Autodesk Inventor part; units mm, degrees
ref_plane "YZ Plane" through (0, 0, 0) normal (1, 0, 0) x (0, 1, 0)
ref_plane "XZ Plane" through (0, 0, 0) normal (0, 1, 0) x (-1, 0, 0)
ref_plane "XY Plane" through (0, 0, 0) normal (0, 0, 1) x (1, 0, 0)
sketch "Sketch1" plane through (0, 0, 0) normal (0, 1, 0) x (-1, 0, 0)
  line L0 (0, 0) -> (400, 0)
  line L1 (400, 0) -> (400, -100)
  line L2 (400, -100) -> (0, -100)
  line L3 (0, -100) -> (0, 0)
  line L4 (320, -103) -> (320, -100)
  line L5 (80, -103) -> (80, -100)
  line L6 (240, -100) -> (240, -103)
  line L7 (160, -103) -> (160, -100)
  line L8 (400, -25) -> (400, -50)
  line L9 (400, -50) -> (403, -50)
  line L10 (200, 0) -> (200, -100) construction
  line L11 (0, 0) -> (0, -100)
  line L12 (-3, -25) -> (0, -25)
  line L13 (0, -25) -> (0, -50)
  line L14 (0, -50) -> (-3, -50)
  line L15 (-3, -75) -> (0, -75)
  line L16 (320, -103) -> (240, -103)
  line L17 (160, -103) -> (80, -103)
  line L18 (0, -100) -> (-3, -100)
  line L19 (-3, -100) -> (-3, -75)
  line L20 (-3, -50) -> (-3, -25)
  line L21 (400, 0) -> (0, 0)
  line L22 (400, -100) -> (400, 0)
  line L23 (403, -75) -> (400, -75)
  line L24 (400, -50) -> (403, -50)
  line L25 (400, -25) -> (400, -50)
  line L26 (403, -25) -> (400, -25)
  line L27 (400, 0) -> (400, -100)
  line L28 (403, -100) -> (403, -75)
  line L29 (403, -50) -> (403, -25)
  line L30 (403, -100) -> (400, -100)
  dimension "d0" = 400
  dimension "d1" = 100
  dimension "d7" = 3
  dimension "d8" = 80
  dimension "d11" = 25
  dimension "d12" = 3
extrude "Extrusion1" add sketch "Sketch1" along normal blind 3
properties part number "Lateral sup e inf"
Verification items for the finished model (mm, model axes). Coordinates: 2 decimals unless noted, no trailing zeros. Loops run counter-clockwise (first coordinate to the right, second up) from the corner with the lowest first, then second, coordinate; pieces in that order, holes last. Notation, with made-up numbers: (-1.75, -23.5) - (2.25, -23.5) arc R17 ccw to (2.25, -3.5) - close; hole circle Ø2 at (60, 26). An arc over 180 degrees is marked (long way). Put each result on its own line as item: value.
Item 1: Scan lines: line 1 along X through (y, z) = (0.75, -65); line 2 along Z through (x, y) = (-166, 2.1). Record each from-to range of solid material in increasing order.
Conclusion:
line 1: x = -400 to 0
line 2: z = -100 to 0
Item 2: Section check A-A (y = 2.45). Enter the section's corners in (x, z), then the cut area to 3 significant figures.
Conclusion:
outline: (-403, -100) - (-320, -100) - (-320, -103) - (-240, -103) - (-240, -100) - (-160, -100) - (-160, -103) - (-80, -103) - (-80, -100) - (3, -100) - (3, -75) - (0, -75) - (0, -50) - (3, -50) - (3, -25) - (0, -25) - (0, 0) - (-400, 0) - (-400, -25) - (-403, -25) - (-403, -50) - (-400, -50) - (-400, -75) - (-403, -75) - close
area: 40,800 mm2
Item 3: Gauge pin test, flat ends, axial feed: pin 1 Ø0.9 at (x, y) = (-193.5, 1) entering from -Z; pin 2 Ø0.9 at (x, y) = (1.5, 1) entering from +Z. Record the tip position at first contact, or that the pin passes through.
Conclusion:
pin 1: stops at z = -100
pin 2: stops at z = -25
Item 4: Section check B-B (x = -36). Enter the section's corners in (y, z).
Conclusion:
outline: (0, -100) - (3, -100) - (3, 0) - (0, 0) - close
